For this review, take the finished solid that the model builds, in its own axes (mm). Face numbers are marked on the shaded views. A direction names the side the tool comes from. Round coordinates to 2 decimals unless told otherwise and drop trailing zeros. Loops run counter-clockwise (first coordinate to the right, second up) from the corner with the lowest first, then second, coordinate; pieces in that order, holes last. Notation, with made-up numbers: (29.25, 59.5) -> (52.25, 59.5) arc R34 ccw to (52.25, 90.5) -> close; hole circle Ø2 at (51.25, -35.75). An arc over 180 degrees is marked (long way). Write each question's results on one line, items separated by ' | '.
Autodesk Inventor part; units mm, degrees
ref_plane "YZ Plane" through (0, 0, 0) normal (1, 0, 0) x (0, 1, 0)
ref_plane "XZ Plane" through (0, 0, 0) normal (0, 1, 0) x (-1, 0, 0)
ref_plane "XY Plane" through (0, 0, 0) normal (0, 0, 1) x (1, 0, 0)
sketch "Sketch1" plane through (0, 0, 0) normal (0, 1, 0) x (-1, 0, 0)
  line L0 (-12, 16) -> (60, 16)
  line L1 (60, 16) -> (60, -30)
  line L2 (60, -30) -> (30, -30)
  line L3 (30, -30) -> (30, -60)
  line L4 (30, -60) -> (-12, -60)
  line L5 (-12, -60) -> (-12, 16)
  dimension "d0" = 72
  dimension "d1" = 46
  dimension "d2" = 30
  dimension "d3" = 30
  dimension "d4" = 42
extrude "Extrusion1" add sketch "Sketch1" along normal blind 15
sketch "Sketch13" plane through (0, 15, 0) normal (0, 1, 0) x (1, 0, 0)
  circle A0 centre (6.5, -10.5) radius 3.75
  circle A1 centre (-24.5, -10.5) radius 3.75
  circle A2 centre (6.5, 20.5) radius 3.75
  circle A3 centre (-24.5, 20.5) radius 3.75
  line L0 (-60, -16) -> (12, -16)
  point P0 (0, 0)
  dimension "d57" = 7.5
  dimension "d58" = 7.5
  dimension "d59" = 7.5
  dimension "d60" = 7.5
  dimension "d68" = 5.5
  dimension "d69" = 31
extrude "Extrusion7" cut sketch "Sketch13" against normal blind 4
sketch "Sketch14" plane through (6.5, 11, 10.5) normal (0, 1, 0) x (1, 0, 0)
  circle A0 centre (0, 0) radius 1.5
  circle A1 centre (-31, 0) radius 1.5
  circle A2 centre (0, 31) radius 3.75
  circle A3 centre (0, 31) radius 1.5
  circle A4 centre (-31, 31) radius 1.5
  point P0 (-6.5, 10.5)
  dimension "d63" = 3
  dimension "d64" = 3
  dimension "d65" = 3
extrude "Extrusion8" cut sketch "Sketch14" against normal up to next contours A0 | A1 | A3 | A4
sketch "Sketch15" plane through (0, 0, 0) normal (0, -1, 0) x (1, 0, 0)
  circle A0 centre (-45, -15) radius 3
  circle A1 centre (-9, -40) radius 1.5
  line L0 (-30, -60) -> (12, -60)
  point P0 (0, 0)
  dimension "d72" = 6
  dimension "d73" = 3
  dimension "d89" = 20
extrude "Extrusion10" cut sketch "Sketch15" against normal up to next
sketch "Sketch16" plane through (0, 0, 0) normal (0, -1, 0) x (1, 0, 0)
  circle A0 centre (-9, -5) radius 7
  point P0 (0, 0)
  dimension "d79" = 14
extrude "Extrusion11" cut sketch "Sketch16" against normal blind 4
sketch "Sketch17" plane through (0, 0, 0) normal (0, -1, 0) x (1, 0, 0)
  line L0 (12, 16) -> (-31, 16)
  line L1 (-31, 16) -> (-31, -27)
  line L2 (-31, -27) -> (12, -27)
  line L3 (12, -27) -> (12, 16)
  point P0 (0, 0)
  dimension "d82" = 43
  dimension "d83" = 43
extrude "Extrusion12" cut sketch "Sketch17" against normal blind 10
sketch "Sketch18" plane through (0, 10, 0) normal (0, -1, 0) x (1, 0, 0)
  circle A0 centre (-9, -5) radius 7
  point P0 (0, 0)
  dimension "d86" = 14
extrude "Extrusion13" cut sketch "Sketch18" against normal blind 3.5
sketch "Sketch19" plane through (0, 0, 0) normal (0, -1, 0) x (1, 0, 0)
  circle A0 centre (-45, -15) radius 5.5
  point P0 (0, 0)
  dimension "d90" = 11
extrude "Extrusion14" cut sketch "Sketch19" against normal blind 11
sketch "Sketch3" plane through (0, 15, 0) normal (0, 1, 0) x (1, 0, 0)
  point P0 (-45, 15)
properties part number "wooden1" material "Aluminum 6061"
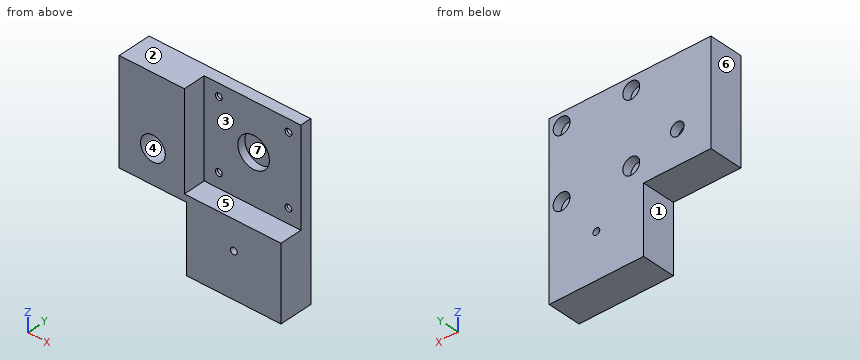
1. Draft analysis for pull direction X (two halves, no side actions). For the marked faces 4, 5, 6 and 7, state which applies: released by +X, released by -X, zero draft, split by the parting line, or undercut.
Values found:
face 4: undercut | face 5: zero draft | face 6: released by -X | face 7: undercut
2. For pin 1 (8 mm diameter, centred on y = 3.5, z = 0, fed in from +X); pin 2 (7 mm diameter, centred on x = 6.5, z = 10.5, fed in from -Y); pin 3 (5 mm diameter, centred on x = -35, y = 4, fed in from -Z), all flat-tipped, find the tip position at first contact; note any pin that passes through.
Values found:
pin 1: stops at x = -31 | pin 2: stops at y = 10 | pin 3: stops at z = -30
3. Consider section D-D (z = -13). State the section outline as (x, y) points.
Values found:
outline: (-60, 0) -> (-50.12, 0) -> (-50.12, 11) -> (-47.24, 11) -> (-47.24, 15) -> (-60, 15) -> close; (-42.76, 11) -> (-39.88, 11) -> (-39.88, 0) -> (-31, 0) -> (-31, 10) -> (12, 10) -> (12, 15) -> (-42.76, 15) -> close
4. Tool access review of the marked faces 1, 2 and 3: name each direction out of +Z, -Z, +X, -X, +Y, -Y from which nothing blocks a thin tool from reaching the whole face with its end or side.
Values found:
face 1: -Z, -X, +Y, -Y | face 2: +Z, +X, -X, +Y, -Y | face 3: +Z, +X, -Y
5. To check wall thickness, follow probe 1 along Z at (x, y) = (-24.5, 10.3); probe 2 along X at (y, z) = (10.55, 10.5); probe 3 along X at (y, z) = (13.85, 10.5). State the ranges of each line that lie inside material, in increasing order.
Values found:
probe 1: z = -60 to -22, -19 to 9, 12 to 16 | probe 2: x = -60 to -26, -23 to 5, 8 to 12 | probe 3: x = -60 to -28.25, -20.75 to 2.75, 10.25 to 12
6. Consider section C-C (y = 2.75). State the section outline as (x, z) points, plus the area to 3 significant figures.
Values found:
outline: (-60, -30) -> (-30, -30) -> (-30, -60) -> (12, -60) -> (12, -27) -> (-31, -27) -> (-31, 16) -> (-60, 16) -> close; hole circle Ø11 at (-45, -15); hole circle Ø3 at (-9, -40) | area: 2,620 mm2
7. Consider section B-B (x = -9). State the section outline as (y, z) points, plus the area to 3 significant figures.
Values found:
outline: (0, -60) -> (15, -60) -> (15, -41.5) -> (0, -41.5) -> close; (0, -38.5) -> (15, -38.5) -> (15, 16) -> (10, 16) -> (10, 2) -> (13.5, 2) -> (13.5, -12) -> (10, -12) -> (10, -27) -> (0, -27) -> close | area: 616 mm2
8. Consider section A-A (z = 10.5). State the section outline as (x, y) points, plus the area to 3 significant figures.
Values found:
outline: (-60, 0) -> (-31, 0) -> (-31, 10) -> (-26, 10) -> (-26, 11) -> (-28.25, 11) -> (-28.25, 15) -> (-60, 15) -> close; (-23, 10) -> (5, 10) -> (5, 11) -> (2.75, 11) -> (2.75, 15) -> (-20.75, 15) -> (-20.75, 11) -> (-23, 11) -> close; (8, 10) -> (12, 10) -> (12, 15) -> (10.25, 15) -> (10.25, 11) -> (8, 11) -> close | area: 584 mm2
